The model under review builds one solid part; all positions refer to its coordinate system, in mm. Face numbers are marked on the shaded views. A direction names the side the tool comes from. Coordinates: 2 decimals unless noted, no trailing zeros. Loops run counter-clockwise (first coordinate to the right, second up) from the corner with the lowest first, then second, coordinate; pieces in that order, holes last. Notation, with made-up numbers: (39, 47.25) - (77, 47.25) arc R12 ccw to (77, 70.25) - close; hole circle Ø1 at (30.5, -17). An arc over 180 degrees is marked (long way). One line per item, written item: value. Start each with the question number.
1. We need section C-C, the plane z = 28. Give the boundary of the cut face in (x, y), then the cut area to 3 significant figures.
2. We need section D-D, the plane x = -17.5. Give the boundary of the cut face in (y, z), then the cut area to 3 significant figures.
3. Insertion check: P1, Ø12, axis at x = -48.5, y = 11.5, coming from the +Z side; P2, Ø3, axis at y = 12.7, z = 38.43, coming from the +X side; P3, Ø7.5, axis at x = -34, y = 6.5, coming from the +Z side; P4, Ø6, axis at x = -46.5, y = 8, coming from the +Z side. Each pin has a flat end and moves straight along its axis. Give the tip position at first contact, or say it passes through.
4. We need section B-B, the plane y = 14. Give the boundary of the cut face in (x, z).
5. Mouldability with a two-part tool opening along X and no side actions: class the marked faces 1, 2, 3 and 4 as +X half, -X half, draft (parallel to the pull), parting line (faces both ways), or undercut.
6. For the marked faces 5, 6 and 7, list the 3-axis set-ups (+Z, -Z, +X, -X, +Y, -Y) from which the entire face can be reached by the end or side of a thin tool; tool diameter is ignored.
7. We need section A-A, the plane z = 4. Give the boundary of the cut face in (x, y).
8. To check wall thickness, follow line 1 (X direction, y = 18.25, z = 7.5); line 2 (Z direction, x = -37.25, y = 12.7); line 3 (X direction, y = 8.75, z = 10). State the ranges of each line that lie inside material, in increasing order.
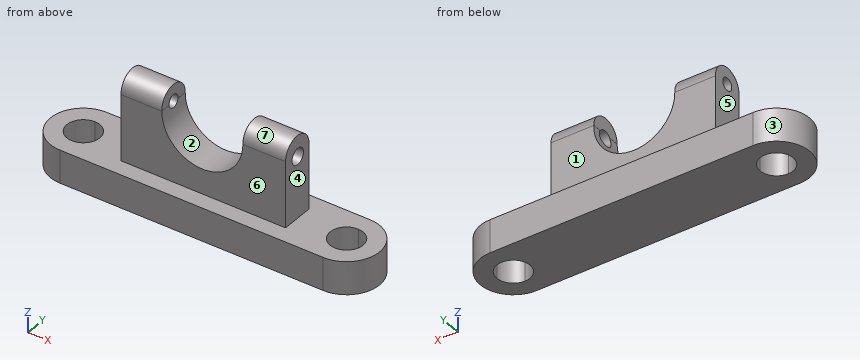
from build123d import *

# Parameters (mm, degrees)
F1_DEPTH  = 12.7
F2_W      = 63.5
F2_H      = 12.7
F3_DEPTH  = 25.4
F5_DEPTH  = 25.4
F8_DEPTH  = 15.7226
F9_DEPTH  = 16.51
F11_R     = 3.127999
F12_DEPTH = 25.4
F10_R     = 2.429756
F13_DEPTH = 25.4


with BuildPart() as f1:
    # F0 (on Top) → F1 (new body)
    with BuildSketch(Plane.XY):
        with BuildLine():
            Line((35.525675, 25.4), (-66.074325, 25.4))
            Line((-66.074325, 25.4), (-66.074325, 19.05))
            ThreePointArc((-66.074325, 19.05), (-61.584197, 17.190128), (-59.724325, 12.7))
            ThreePointArc((-59.724325, 12.7), (-61.584197, 8.209872), (-66.074325, 6.35))
            Line((-66.074325, 6.35), (-66.074325, 0))
            Line((-66.074325, 0), (35.525675, 0))
            Line((35.525675, 0), (35.525675, 6.35))
            ThreePointArc((35.525675, 6.35), (29.175675, 12.7), (35.525675, 19.05))
            Line((35.525675, 19.05), (35.525675, 25.4))
        make_face()
        Polygon((-47.024325, 6.35), (-47.024325, 12.7), (-47.024325, 19.05), (16.475675, 19.05), (16.475675, 6.35), align=None, mode=Mode.SUBTRACT)
        with BuildLine():
            Line((-66.074325, 19.05), (-66.074325, 25.4))
            ThreePointArc((-66.074325, 25.4), (-78.774325, 12.7), (-66.074325, 0))
            Line((-66.074325, 0), (-66.074325, 6.35))
            ThreePointArc((-66.074325, 6.35), (-72.424325, 12.7), (-66.074325, 19.05))
        make_face()
        with BuildLine():
            ThreePointArc((35.525675, 0), (48.225675, 12.7), (35.525675, 25.4))
            Line((35.525675, 25.4), (35.525675, 19.05))
            ThreePointArc((35.525675, 19.05), (40.015803, 17.190128), (41.875675, 12.7))
            ThreePointArc((41.875675, 12.7), (40.015803, 8.209872), (35.525675, 6.35))
            Line((35.525675, 6.35), (35.525675, 0))
        make_face()
        Polygon((-47.024325, 19.05), (-47.024325, 12.7), (-47.024325, 6.35), (16.475675, 6.35), (16.475675, 19.05), align=None)
    extrude(amount=F1_DEPTH)

    # F2 (on face) → F3 (join)
    with BuildSketch(Plane.XY.offset(12.7)):
        with Locations((-15.274325, 12.7)):
            Rectangle(F2_W, F2_H)
    extrude(amount=F3_DEPTH)

    # F4 (on face) → F5 (cut)
    with BuildSketch(Plane.XZ.offset(-6.35)):
        with BuildLine():
            Line((0, 38.1), (-31.290911, 38.1))
            ThreePointArc((-31.290911, 38.1), (-15.645456, 22.243986), (0, 38.1))
        make_face()
    extrude(amount=-F5_DEPTH, mode=Mode.SUBTRACT)

    # F7 (on face) → F8 (join)
    with BuildSketch(Plane(origin=(-47.024325, 0, 0), x_dir=(0, -1, 0), z_dir=(-1, 0, 0))):
        with BuildLine():
            Line((-19.05, 38.1), (-6.35, 38.1))
            ThreePointArc((-6.35, 38.1), (-12.7, 44.788843), (-19.05, 38.1))
        make_face()
    extrude(amount=-F8_DEPTH)

    # F6 (on face) → F9 (join)
    with BuildSketch(Plane.YZ.offset(16.475675)):
        with BuildLine():
            Line((6.35, 38.1), (19.05, 38.1))
            ThreePointArc((19.05, 38.1), (12.7, 44.45), (6.35, 38.1))
        make_face()
    extrude(amount=-F9_DEPTH)

    # F11 (on face) → F12 (cut)
    with BuildSketch(Plane.YZ.offset(16.475675)):
        with Locations((12.986762, 36.340035)):
            Circle(F11_R)
    extrude(amount=-F12_DEPTH, mode=Mode.SUBTRACT)

    # F10 (on face) → F13 (cut)
    with BuildSketch(Plane(origin=(-47.024325, 0, 0), x_dir=(0, -1, 0), z_dir=(-1, 0, 0))):
        with Locations((-12.7, 38.430261)):
            Circle(F10_R)
    extrude(amount=-F13_DEPTH, mode=Mode.SUBTRACT)


solid = f1.part
Findings below:
1. outline: (-47.02, 6.35) - (-27.77, 6.35) - (-27.77, 19.05) - (-47.02, 19.05) - close; (-3.52, 6.35) - (16.48, 6.35) - (16.48, 19.05) - (-3.52, 19.05) - close
1. area: 498 mm2
2. outline: (0, 0) - (25.4, 0) - (25.4, 12.7) - (19.05, 12.7) - (19.05, 22.35) - (6.35, 22.35) - (6.35, 12.7) - (0, 12.7) - close
2. area: 445 mm2
3. P1: z = 44.79
3. P2: x = 16.48
3. P3: z = 44.3
3. P4: z = 44.56
4. outline: (-78.71, 0) - (-72.29, 0) - (-72.29, 12.7) - (-78.71, 12.7) - close; (-59.86, 0) - (29.31, 0) - (29.31, 12.7) - (16.48, 12.7) - (16.48, 33.38) - (-0.66, 33.38) arc R15.65 cw to (-31.22, 36.38) - (-47.02, 36.38) - (-47.02, 12.7) - (-59.86, 12.7) - close; (-47.02, 40.48) - (-31.3, 40.48) - (-31.3, 44.65) - (-47.02, 44.65) - close; (-0.03, 39.3) - (16.48, 39.3) - (16.48, 44.32) - (-0.03, 44.32) - close; (41.74, 0) - (48.16, 0) - (48.16, 12.7) - (41.74, 12.7) - close
5. face 1: draft
5. face 2: undercut
5. face 3: -X half
5. face 4: +X half
6. face 5: +Z, -X, +Y, -Y
6. face 6: +Z, +X, -X, -Y
6. face 7: +Z, +X
7. outline: (-66.07, 0) - (35.53, 0) arc R12.7 ccw to (35.53, 25.4) - (-66.07, 25.4) arc R12.7 ccw to start; hole circle Ø12.7 at (-66.07, 12.7); hole circle Ø12.7 at (35.53, 12.7)
8. line 1: -77.5 to -69.16, -62.99 to 32.44, 38.61 to 46.95
8. line 2: 0 to 36, 40.86 to 44.79
8. line 3: -78.14 to -71.05, -61.1 to 30.55, 40.5 to 47.6
